The drawing under review shows one solid part. Ordinate dimensions are in mm from its lowest x, y, z. A direction names the side the tool comes from. Coordinates: 2 decimals unless noted, no trailing zeros. Write each loop counter-clockwise with the first axis right and the second up, starting at its lowest first coordinate (ties: lowest second). Pieces come first, ordered by that corner, then holes. Notation, with made-up numbers: M -16,-14 L 1,-14 A13 cw 1,5 Z; hole C 81.5,-27 d1. An arc over 180 degrees is marked long. Write each question's results on one line, items separated by ' | '. Start each with the question number.
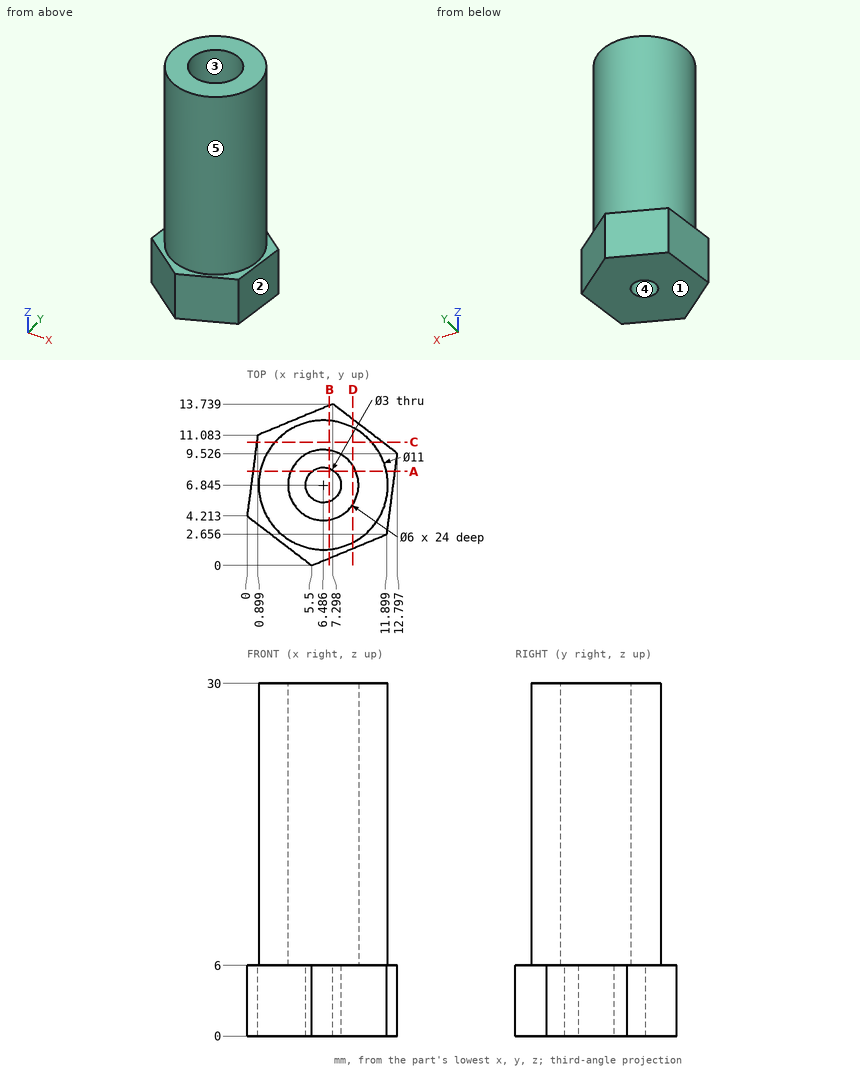
Item 1: We need section C-C on y = 10.5. State the section outline as (x, z) points.
Item 2: Insertion check: pin 1 Ø4 at (x, y) = (6.49, 6.85) entering from +Z; pin 2 Ø2 at (x, z) = (10.5, 8) entering from -Y (1 decimal); pin 3 Ø6 at (x, z) = (6.5, 22) entering from +Y (1 decimal). Each pin has a flat end and moves straight along its axis. Give the tip position at first contact, or say it passes through.
Item 3: We need section A-A on y = 8. State the section outline as (x, z) points (1 decimal).
Item 4: We need section D-D on x = 9. State the section outline as (y, z) points (1 decimal).
Item 5: Draft analysis for pull direction Y (two halves, no side actions). For the marked faces 1, 2 and 3, state which applies: released by +Y, released by -Y, zero draft, split by the parting line, or undercut.
Item 6: We need section B-B on x = 7. State the section outline as (y, z) points (1 decimal).
Item 7: For the marked faces 4 and 5, list the 3-axis set-ups (+Z, -Z, +X, -X, +Y, -Y) from which the entire face can be reached by the end or side of a thin tool; tool diameter is ignored.
Item 8: Wall thickness on L1, parallel to Z at x = 8.75, y = 5; L2, parallel to Y at x = 4.5, z = 11.5 (1 decimal); L3, parallel to X at y = 4.5, z = 10.25 (1 decimal): over which ranges is each line inside the solid? List them lowest first.
Answer:
1) outline: M 0.82,0 L 11.53,0 L 11.53,6 L 10.6,6 L 10.6,30 L 2.38,30 L 2.38,6 L 0.82,6 Z
2) pin 1: stops at z = 6 | pin 2: stops at y = 2.2 | pin 3: stops at y = 12.3
3) outline: M 0.5,0 L 5.5,0 L 5.5,6 L 3.7,6 L 3.7,30 L 1.1,30 L 1.1,6 L 0.5,6 Z; M 7.4,0 L 12.6,0 L 12.6,6 L 11.9,6 L 11.9,30 L 9.3,30 L 9.3,6 L 7.4,6 Z
4) outline: M 1.5,0 L 12.4,0 L 12.4,6 L 11.7,6 L 11.7,30 L 8.5,30 L 8.5,6 L 5.2,6 L 5.2,30 L 2,30 L 2,6 L 1.5,6 Z
5) face 1: zero draft | face 2: released by -Y | face 3: undercut
6) outline: M 0.6,0 L 5.4,0 L 5.4,6 L 3.9,6 L 3.9,30 L 1.4,30 L 1.4,6 L 0.6,6 Z; M 8.3,0 L 13.6,0 L 13.6,6 L 12.3,6 L 12.3,30 L 9.8,30 L 9.8,6 L 8.3,6 Z
7) face 4: +Z, -Z | face 5: +Z
8) L1: z = 0 to 6 | L2: y = 1.7 to 4.6, 9.1 to 12 | L3: x = 1.5 to 4.6, 8.4 to 11.5
